from build123d import *

# Parameters (mm, degrees)
BOSS_EXTRUDE2_DEPTH = 34
SKETCH5_W           = 50
SKETCH5_H           = 20
CUT_EXTRUDE1_DEPTH  = 8.5
SKETCH6_W           = 50
SKETCH6_H           = 20
CUT_EXTRUDE2_DEPTH  = 8.5
SKETCH7_W           = 52.006330756
SKETCH7_H           = 21.627895193
CUT_EXTRUDE3_DEPTH  = 87.390073596
CUT_EXTRUDE4_DEPTH  = 101.468874862
SKETCH10_R          = 1.75
CUT_EXTRUDE5_DEPTH  = 10
SKETCH14_W          = 15
SKETCH14_H          = 37
CUT_EXTRUDE8_DEPTH  = 18
SKETCH15_W          = 18
SKETCH15_H          = 15
CUT_EXTRUDE9_DEPTH  = 9
SKETCH16_W          = 13
SKETCH16_H          = 9
CUT_EXTRUDE10_DEPTH = 96.362439231
SKETCH17_R          = 1.75
CUT_EXTRUDE11_DEPTH = 87.390073596


with BuildPart() as part:
    # Sketch4 → Boss-Extrude2 (new body)
    with BuildSketch(Plane.XY):
        with BuildLine():
            Line((-25, -10), (30, -10))
            Line((30, -10), (30, 30.414))
            ThreePointArc((30, 30.414), (22.015013929, 47.178), (30, 63.942))
            Line((30, 63.942), (30, 76.896))
            Line((30, 76.896), (7.747226033, 76.896))
            Line((7.747226033, 76.896), (-25, 10))
            Line((-25, 10), (-25, -10))
        make_face()
    extrude(amount=BOSS_EXTRUDE2_DEPTH)

    # Sketch5 → Cut-Extrude1 (cut)
    with BuildSketch(Plane.XY.offset(34)):
        Polygon((-23.041902294, 14), (7.747226033, 76.896), (20, 76.896), (20, 14), align=None)
        Rectangle(SKETCH5_W, SKETCH5_H)
    extrude(amount=-CUT_EXTRUDE1_DEPTH, mode=Mode.SUBTRACT)

    # Sketch6 → Cut-Extrude2 (cut)
    with BuildSketch(Plane(origin=(0, 0, 0), x_dir=(-1, 0, 0), z_dir=(0, 0, -1))):
        Polygon((23.041902294, 14), (-20, 14), (-20, 76.896), (-7.747226033, 76.896), align=None)
        Rectangle(SKETCH6_W, SKETCH6_H)
    extrude(amount=-CUT_EXTRUDE2_DEPTH, mode=Mode.SUBTRACT)

    # Sketch7 → Cut-Extrude3 (cut, through all)
    with BuildSketch(Plane(origin=(0, 0, 8.5), x_dir=(-1, 0, 0), z_dir=(0, 0, -1))):
        with Locations((1.003165378, -0.813947597)):
            Rectangle(SKETCH7_W, SKETCH7_H)
    extrude(amount=-CUT_EXTRUDE3_DEPTH, mode=Mode.SUBTRACT)

    # Sketch9 → Cut-Extrude4 (cut, through all)
    with BuildSketch(Plane(origin=(30, 0, 0), x_dir=(0, 0, -1), z_dir=(1, 0, 0))):
        with BuildLine():
            Line((-26.615, 9.257), (-7.385, 9.257))
            ThreePointArc((-7.385, 9.257), (-3.487778361, 7.006814103), (-3.488100353, 2.506628222))
            Line((-3.488100353, 2.506628222), (-13.103100353, -14.143371778))
            ThreePointArc((-13.103100353, -14.143371778), (-17, -16.393), (-20.896899647, -14.143371778))
            Line((-20.896899647, -14.143371778), (-30.511899647, 2.506628222))
            ThreePointArc((-30.511899647, 2.506628222), (-30.512221639, 7.006814103), (-26.615, 9.257))
        make_face()
    extrude(amount=-CUT_EXTRUDE4_DEPTH, mode=Mode.SUBTRACT)

    # Sketch10 → Cut-Extrude5 (cut)
    with BuildSketch(Plane.XZ.offset(-10)):
        with Locations(Location((16, 29.5, 0), (0, 0, 270))):
            Circle(SKETCH10_R)
        with Locations(Location((16, 4.5, 0), (0, 0, 270))):
            Circle(SKETCH10_R)
        with Locations(Location((-16, 29.5, 0), (0, 0, 270))):
            Circle(SKETCH10_R)
        with Locations(Location((-16, 4.5, 0), (0, 0, 270))):
            Circle(SKETCH10_R)
    extrude(amount=-CUT_EXTRUDE5_DEPTH, mode=Mode.SUBTRACT)

    # Sketch14 → Cut-Extrude8 (cut)
    with BuildSketch(Plane.ZY.offset(-20)):
        with Locations((17, 58.396)):
            Rectangle(SKETCH14_W, SKETCH14_H)
    extrude(amount=CUT_EXTRUDE8_DEPTH, mode=Mode.SUBTRACT)

    # Sketch15 → Cut-Extrude9 (cut)
    with BuildSketch(Plane(origin=(0, 39.896, 0), x_dir=(1, 0, 0), z_dir=(0, 1, 0))):
        with Locations((11, -17)):
            Rectangle(SKETCH15_W, SKETCH15_H)
    extrude(amount=-CUT_EXTRUDE9_DEPTH, mode=Mode.SUBTRACT)

    # Sketch16 → Cut-Extrude10 (cut, through all)
    with BuildSketch(Plane.ZY.offset(-20)):
        with Locations((17, 35.396)):
            Rectangle(SKETCH16_W, SKETCH16_H)
    extrude(amount=CUT_EXTRUDE10_DEPTH, mode=Mode.SUBTRACT)

    # Sketch17 → Cut-Extrude11 (cut, through all)
    with BuildSketch(Plane.XY.offset(25.5)):
        with Locations((12.5, 35.396)):
            Circle(SKETCH17_R)
    extrude(amount=-CUT_EXTRUDE11_DEPTH, mode=Mode.SUBTRACT)


solid = part.part
Build history of the part. All positions in model axes, mm. A direction names the side the tool comes from. Round coordinates to 2 decimals unless told otherwise and drop trailing zeros. Write each loop counter-clockwise with the first axis right and the second up, starting at its lowest first coordinate (ties: lowest second). Pieces come first, ordered by that corner, then holes. Notation, with made-up numbers: (24.5, 13.25) -> (70.5, 13.25) arc R20 ccw to (70.5, 34.25) -> close; hole circle Ø2 at (73.25, 50.5). An arc over 180 degrees is marked (long way). Write item = value, one per line.
(1) Flat gauge pins, fed straight in: pin 1 (12 mm diameter, centred on y = 56.5, z = 19.5, fed in from +X); pin 2 (1.5 mm diameter, centred on x = 0, y = 30, fed in from -Z); pin 3 (4 mm diameter, centred on x = 27, z = 18, fed in from -Y). Where does each tip first touch, or does it go through?
Answer:
pin_1 = 28.39
pin_2 = 8.5
pin_3 = 9.26
(2) Band-saw the part on C-C (z = 4.5). Give the cut face in (x, y).
Answer:
outline = (-25, 10) -> (-17.75, 10) -> (-17.75, 14) -> (-23.04, 14) -> close; (-14.25, 10) -> (14.25, 10) -> (14.25, 14) -> (-14.25, 14) -> close; (17.75, 10) -> (25, 10) -> (25, 8.21) -> (30, 8.21) -> (30, 30.41) arc R21.59 cw to (30, 63.94) -> (30, 76.9) -> (20, 76.9) -> (20, 14) -> (17.75, 14) -> close; (25, -10) -> (30, -10) -> (30, 0.75) -> (25, 0.75) -> close
(3) Tool access for faces 3 (the face through (2, 52, 17)), 4 (the face through (-1, 14, 30)), 5 (the face through (-2, 14, 4)), 6 (the face through (0, 10, 17)), 7 (the face through (27.54, -3.66, 7.05)): list every direction of +Z, -Z, +X, -X, +Y, -Y with a clear straight run to the whole face (end or side of a thin tool).
Answer:
face_3 = +Y
face_4 = +Z, -X, +Y
face_5 = -Z, -X, +Y
face_6 = +Z, -Z, -X, -Y
face_7 = +X, -X
(4) Band-saw the part on B-B (x = 12.5). Give the cut face in (y, z).
Answer:
outline = (10, 0) -> (14, 0) -> (14, 8.5) -> (33.65, 8.5) -> (33.65, 9.5) -> (30.9, 9.5) -> (30.9, 24.5) -> (33.65, 24.5) -> (33.65, 25.5) -> (14, 25.5) -> (14, 34) -> (10, 34) -> close; (37.15, 8.5) -> (76.9, 8.5) -> (76.9, 9.5) -> (37.15, 9.5) -> close; (37.15, 24.5) -> (76.9, 24.5) -> (76.9, 25.5) -> (37.15, 25.5) -> close
(5) Band-saw the part on A-A (z = 13). Give the cut face in (x, y).
Answer:
outline = (-25, 10) -> (25, 10) -> (25, 9.26) -> (30, 9.26) -> (30, 30.41) arc R21.59 cw to (30, 63.94) -> (30, 76.9) -> (20, 76.9) -> (20, 30.9) -> (-14.77, 30.9) -> close; (-10.37, 39.9) -> (2, 39.9) -> (2, 65.16) -> close
(6) Band-saw the part on D-D (y = 41). Give the cut face in (x, z).
Answer:
outline = (-9.82, 8.5) -> (20, 8.5) -> (20, 0) -> (22.92, 0) -> (22.92, 34) -> (20, 34) -> (20, 25.5) -> (-9.82, 25.5) -> close; hole (2, 9.5) -> (20, 9.5) -> (20, 24.5) -> (2, 24.5) -> close
(7) Two-plate mould, pull along Z, no slides. Class faces 1 (the face through (17.735, 11.972, 4.728)), 2 (the face through (27, -10, 29)): pulls with the +Z half, pulls with the -Z half, needs draft (parallel to the pull), parting line crosses it, or undercut.
Answer:
face_1 = undercut
face_2 = needs draft
(8) Probe L1, parallel to Z at x = 9.5, y = 44; L2, parallel to X at y = 13, z = 4.5; L3, parallel to X at y = 11, z = 4. List the from-to ranges inside material, lowest first.
Answer:
L1 = 8.5 to 9.5, 24.5 to 25.5
L2 = -23.53 to -17.75, -14.25 to 14.25, 17.75 to 30
L3 = -24.51 to -17.68, -14.32 to 14.32, 17.68 to 30
